Read the model definition and answer for the solid it produces. Units are mm, in the model's axes. Face numbers are marked on the shaded views. A direction names the side the tool comes from. Round coordinates to 2 decimals unless told otherwise and drop trailing zeros. Write each loop counter-clockwise with the first axis right and the second up, starting at its lowest first coordinate (ties: lowest second). Pieces come first, ordered by that corner, then holes.
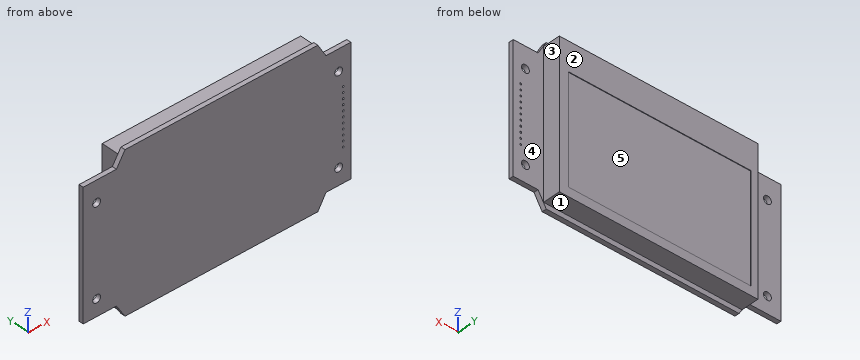
from build123d import *

# Parameters (mm, degrees)
BOSS_EXTRUDE1_DEPTH = 1.6
SKETCH2_R           = 1.397
CUT_EXTRUDE1_DEPTH  = 67.676798076
SKETCH3_W           = 70.612
SKETCH3_H           = 51.435
BOSS_EXTRUDE2_DEPTH = 6.2357
SKETCH4_W           = 65.024
SKETCH4_H           = 38.1
CUT_EXTRUDE2_DEPTH  = 0.2
SKETCH5_R           = 0.3302
CUT_EXTRUDE3_DEPTH  = 67.94863222
LPATTERN1_COUNT     = 11
LPATTERN1_PITCH     = 2


with BuildPart() as part:
    # Sketch1 → Boss-Extrude1 (new body)
    with BuildSketch(Plane(origin=(0, 0, 0), x_dir=(1, 0, 0), z_dir=(0, 1, 0))):
        Polygon((-60.059561589, 21.169974834), (-60.059561589, -23.991225166), (-48.223161589, -23.991225166), (-45.175161589, -28.915125166), (23.404838411, -28.915125166), (26.351238411, -23.991225166), (35.190438411, -23.991225166), (35.190438411, 21.169974834), (26.351238411, 21.169974834), (23.404838411, 26.084874834), (-45.175161589, 26.084874834), (-48.223161589, 21.169974834), align=None)
    extrude(amount=BOSS_EXTRUDE1_DEPTH)

    # Sketch2 → Cut-Extrude1 (cut, through all)
    with BuildSketch(Plane(origin=(0, 1.6, 0), x_dir=(1, 0, 0), z_dir=(0, 1, 0))):
        with Locations(Location((-55.271661589, 15.251774834, 0), (0, 0, 270))):
            Circle(SKETCH2_R)
        with Locations(Location((-55.271661589, -16.498225166, 0), (0, 0, 270))):
            Circle(SKETCH2_R)
        with Locations(Location((30.834338411, -16.498225166, 0), (0, 0, 270))):
            Circle(SKETCH2_R)
        with Locations(Location((30.834338411, 15.251774834, 0), (0, 0, 270))):
            Circle(SKETCH2_R)
    extrude(amount=-CUT_EXTRUDE1_DEPTH, mode=Mode.SUBTRACT)

    # Sketch3 → Boss-Extrude2 (add)
    with BuildSketch(Plane(origin=(0, 1.6, 0), x_dir=(1, 0, 0), z_dir=(0, 1, 0))):
        with Locations((-10.910561589, -1.382625166)):
            Rectangle(SKETCH3_W, SKETCH3_H)
    extrude(amount=BOSS_EXTRUDE2_DEPTH)

    # Sketch4 → Cut-Extrude2 (cut)
    with BuildSketch(Plane(origin=(0, 7.8357, 0), x_dir=(1, 0, 0), z_dir=(0, 1, 0))):
        with Locations((-11.291561589, 2.109874834)):
            Rectangle(SKETCH4_W, SKETCH4_H)
    extrude(amount=-CUT_EXTRUDE2_DEPTH, mode=Mode.SUBTRACT)

    # Sketch5 → Cut-Extrude3 (cut, through all)
    with BuildSketch(Plane(origin=(0, 1.6, 0), x_dir=(1, 0, 0), z_dir=(0, 1, 0))):
        with Locations(Location((32.490438411, 9.299974834, 0), (0, 0, 270))):
            Circle(SKETCH5_R)
    cut_extrude3 = extrude(amount=-CUT_EXTRUDE3_DEPTH, mode=Mode.SUBTRACT)

    # LPattern1: Cut-Extrude3 ×11
    with Locations(*[(0, 0, i * LPATTERN1_PITCH) for i in range(1, LPATTERN1_COUNT)]):
        add(cut_extrude3, mode=Mode.SUBTRACT)


solid = part.part
Q1. Section B-B (z = 20.5) is taken. Determine the outline of the cut face in (x, y).
Verdict:
outline: (-60.06, 0) - (35.19, 0) - (35.19, 1.6) - (24.4, 1.6) - (24.4, 7.84) - (-46.22, 7.84) - (-46.22, 1.6) - (-60.06, 1.6) - close
Q2. Section C-C (x = -1.5) is taken. Determine the outline of the cut face in (y, z), then the cut area to 3 significant figures.
Verdict:
outline: (0, -26.08) - (1.6, -26.08) - (1.6, -24.33) - (7.84, -24.33) - (7.84, -21.16) - (7.64, -21.16) - (7.64, 16.94) - (7.84, 16.94) - (7.84, 27.1) - (1.6, 27.1) - (1.6, 28.92) - (0, 28.92) - close
area: 401 mm2
Q3. Straight lines are drawn through the part: probe 1 along X at (y, z) = (6, 5); probe 2 along Y at (x, z) = (-14, -10.5); probe 3 along Y at (x, z) = (-52, 19.5). For each, find the intervals that lie inside material, in ascending order.
Verdict:
probe 1: x = -46.22 to 24.4
probe 2: y = 0 to 7.64
probe 3: y = 0 to 1.6
Q4. Section A-A (z = -15) is taken. Determine the outline of the cut face in (x, y), then the cut area to 3 significant figures.
Verdict:
outline: (-60.06, 0) - (-56.65, 0) - (-56.65, 1.6) - (-60.06, 1.6) - close; (-53.9, 0) - (29.46, 0) - (29.46, 1.6) - (24.4, 1.6) - (24.4, 7.84) - (21.22, 7.84) - (21.22, 7.64) - (-43.8, 7.64) - (-43.8, 7.84) - (-46.22, 7.84) - (-46.22, 1.6) - (-53.9, 1.6) - close; (32.21, 0) - (35.19, 0) - (35.19, 1.6) - (32.21, 1.6) - close
area: 571 mm2
Q5. Which of the six approach directions +Z, -Z, +X, -X, +Y, -Y give full straight-line access (tool end or side, diameter ignored) to the marked faces 1 and 2?
Verdict:
face 1: -Z, +X, -X, +Y
face 2: +Z, -Z, +X, -X, +Y
Q6. Section D-D (y = 3.5) is taken. Determine the outline of the cut face in (x, z).
Verdict:
outline: (-46.22, -24.33) - (24.4, -24.33) - (24.4, 27.1) - (-46.22, 27.1) - close
Q7. Flat-ended cylindrical pins translate along their axes: pin 1 Ø3 at (y, z) = (4.5, -4) entering from -X; pin 2 Ø1.5 at (x, z) = (-17, -2) entering from -Y; pin 3 Ø8 at (x, z) = (13.5, 1.5) entering from +Y; pin 4 Ø1.9 at (x, y) = (-24.5, 4) entering from +Z. Find the tip coordinate at first contact, or state that the pin passes through.
Verdict:
pin 1: stops at x = -46.22
pin 2: stops at y = 0
pin 3: stops at y = 7.64
pin 4: stops at z = 27.1
Q8. Determine the mould class of the marked faces 3, 4 and 5 for opening direction X: pulls with the +X half, pulls with the -X half, needs draft (parallel to the pull), parting line crosses it, or undercut.
Verdict:
face 3: pulls with the +X half
face 4: needs draft
face 5: undercut
